from build123d import *

# Parameters (mm, degrees)
SKETCH_1_W          = 48
SKETCH_1_H          = 17
EXTRUDE_1_DEPTH     = 2.5
SKETCH_2_W          = 48
SKETCH_2_H          = 5
EXTRUDE_2_DEPTH     = 16
SKETCH_3_R          = 1.5
CUT_EXTRUDE_1_DEPTH = 20
FILLET_1_R          = 6
SKETCH_4_R          = 1.5
CUT_EXTRUDE_2_DEPTH = 20


with BuildPart() as part:
    # 草图1 → 凸台-拉伸1 (new body)
    with BuildSketch(Plane(origin=(0, 0, 0), x_dir=(1, 0, 0), z_dir=(0, 1, 0))):
        Rectangle(SKETCH_1_W, SKETCH_1_H)
    extrude(amount=EXTRUDE_1_DEPTH)

    # 草图2 → 凸台-拉伸2 (add)
    with BuildSketch(Plane(origin=(0, 2.5, 0), x_dir=(1, 0, 0), z_dir=(0, 1, 0))):
        with Locations((0, -6)):
            Rectangle(SKETCH_2_W, SKETCH_2_H)
    extrude(amount=EXTRUDE_2_DEPTH)

    # 草图3 → 切除-拉伸1 (cut)
    with BuildSketch(Plane(origin=(0, 2.5, 0), x_dir=(1, 0, 0), z_dir=(0, 1, 0))):
        with Locations(Location((18.75, 3, 0), (0, 0, 270))):
            Circle(SKETCH_3_R)
        with Locations(Location((-18.75, 3, 0), (0, 0, 270))):
            Circle(SKETCH_3_R)
    extrude(amount=-CUT_EXTRUDE_1_DEPTH, mode=Mode.SUBTRACT)

    # 圆角1
    fillet_1_edges = [part.edges().sort_by_distance(p)[0] for p in [
        (24, 18.5, 6),
        (-24, 18.5, 6),
        (-24, 1.25, -8.5),
        (24, 1.25, -8.5),
    ]]
    fillet(fillet_1_edges, radius=FILLET_1_R)

    # 草图4 → 切除-拉伸2 (cut)
    with BuildSketch(Plane(origin=(0, 0, 3.5), x_dir=(-1, 0, 0), z_dir=(0, 0, -1))):
        with Locations((17.5, 12)):
            Circle(SKETCH_4_R)
        with Locations((-17.5, 12)):
            Circle(SKETCH_4_R)
    extrude(amount=-CUT_EXTRUDE_2_DEPTH, mode=Mode.SUBTRACT)


solid = part.part
Part model, mm, in its own coordinate system. A direction names the side the tool comes from. Round coordinates to 2 decimals unless told otherwise and drop trailing zeros. Loops run counter-clockwise (first coordinate to the right, second up) from the corner with the lowest first, then second, coordinate; pieces in that order, holes last. Notation, with made-up numbers: (-18, -19.75) - (6, -19.75) arc R13 cw to (6, -7.75) - close; hole circle Ø9 at (22.5, -29). An arc over 180 degrees is marked (long way). Answer as a JSON object with one key per item and string values.
Item 1: Band-saw the part on A-A on y = 12. List the corners of the cut face in (x, z), plus the area to 3 significant figures.
Output:
{"outline": "(-24, 3.5) - (-19, 3.5) - (-19, 8.5) - (-24, 8.5) - close; (-16, 3.5) - (16, 3.5) - (16, 8.5) - (-16, 8.5) - close; (19, 3.5) - (24, 3.5) - (24, 8.5) - (19, 8.5) - close", "area": "210 mm2"}
Item 2: Band-saw the part on B-B on x = -15. List the corners of the cut face in (y, z), plus the area to 4 significant figures.
Output:
{"outline": "(0, -8.5) - (2.5, -8.5) - (2.5, 3.5) - (18.5, 3.5) - (18.5, 8.5) - (0, 8.5) - close", "area": "122.5 mm2"}
Item 3: Wall check: L1, parallel to Z at x = 6.5, y = 15.25; L2, parallel to Z at x = 18, y = 1.75; L3, parallel to Y at x = 18.5, z = 0. Give the ranges that are in metal, low to high.
Output:
{"L1": "3.5 to 8.5", "L2": "-8.5 to -4.3, -1.7 to 8.5", "L3": "0 to 2.5"}
Item 4: Pull direction Z, two halves, no side cores. Call faces 1 (the face through (-22.289, 1.268, -6.696)), 2 (the face through (-17.485, 1.268, -2.194)), 3 (the face through (20.015, 1.268, -2.194)), 4 (the face through (-22.289, 16.696, 5.965)): pulls with the +Z half, pulls with the -Z half, needs draft (parallel to the pull), parting line crosses it, or undercut.
Output:
{"face 1": "pulls with the -Z half", "face 2": "undercut", "face 3": "undercut", "face 4": "needs draft"}
Item 5: Band-saw the part on D-D on y = 9.5. List the corners of the cut face in (x, z).
Output:
{"outline": "(-24, 3.5) - (24, 3.5) - (24, 8.5) - (-24, 8.5) - close"}
Item 6: Pin check, flat tips, straight feed: pin 1 (2 mm diameter, centred on x = -19, y = 13.5, fed in from -Z); pin 2 (6 mm diameter, centred on x = -8, z = -1, fed in from +Y). Stop position of each tip, or through.
Output:
{"pin 1": "z = 3.5", "pin 2": "y = 2.5"}
Item 7: Band-saw the part on C-C on z = -3. List the corners of the cut face in (x, y).
Output:
{"outline": "(-23.98, 0) - (-20.25, 0) - (-20.25, 2.5) - (-23.98, 2.5) - close; (-17.25, 0) - (17.25, 0) - (17.25, 2.5) - (-17.25, 2.5) - close; (20.25, 0) - (23.98, 0) - (23.98, 2.5) - (20.25, 2.5) - close"}
Item 8: Tool access for faces 5 (the face through (0, 18.5, 6)), 6 (the face through (0, 10, 3.5)): list every direction of +Z, -Z, +X, -X, +Y, -Y with a clear straight run to the whole face (end or side of a thin tool).
Output:
{"face 5": "+Z, -Z, +X, -X, +Y", "face 6": "-Z, +X, -X, +Y"}
